```python
from build123d import *

# Parameters (mm, degrees)
SKETCH1_R           = 46.5
SKETCH1_R_2         = 36
BOSS_EXTRUDE1_DEPTH = 6.25
SKETCH4_R           = 36
SKETCH4_R_2         = 34
BOSS_EXTRUDE2_DEPTH = 3.5
SKETCH3_R           = 1.75
CUT_EXTRUDE1_DEPTH  = 67.938404522
CIRPATTERN1_COUNT   = 8


with BuildPart() as part:
    # Sketch1 → Boss-Extrude1 (new, symmetric)
    with BuildSketch(Plane.XY):
        Circle(SKETCH1_R)
        Circle(SKETCH1_R_2, mode=Mode.SUBTRACT)
    extrude(amount=BOSS_EXTRUDE1_DEPTH, both=True)

    # Sketch4 → Boss-Extrude2 (add)
    with BuildSketch(Plane.XY.offset(-6.25)):
        Circle(SKETCH4_R)
        Circle(SKETCH4_R_2, mode=Mode.SUBTRACT)
    extrude(amount=BOSS_EXTRUDE2_DEPTH)

    # Sketch3 → Cut-Extrude1 (cut, through all)
    with BuildSketch(Plane.XY.offset(6.25)):
        with Locations((0, 40.25)):
            Circle(SKETCH3_R)
    cut_extrude1 = extrude(amount=-CUT_EXTRUDE1_DEPTH, mode=Mode.SUBTRACT)

    # CirPattern1: Cut-Extrude1 ×8 about axis
    cirpattern1_axis = Axis((0, 0, 0), (0, 0, 1))
    for i in range(1, CIRPATTERN1_COUNT):
        add(cut_extrude1.rotate(cirpattern1_axis, i * 360 / CIRPATTERN1_COUNT), mode=Mode.SUBTRACT)


solid = part.part
```
Work out the finished part from the listing and answer in its coordinate system (mm). A direction names the side the tool comes from. Coordinates: 2 decimals unless noted, no trailing zeros. Write each loop counter-clockwise with the first axis right and the second up, starting at its lowest first coordinate (ties: lowest second). Pieces come first, ordered by that corner, then holes. Notation, with made-up numbers: (60.25, -11.5) - (116.25, -11.5) arc R15 ccw to (116.25, 13.5) - close; hole circle Ø2 at (-16.5, -11.75). An arc over 180 degrees is marked (long way). Answer as a JSON object with one key per item and string values.
Q1. Which of the six approach directions +Z, -Z, +X, -X, +Y, -Y give full straight-line access (tool end or side, diameter ignored) to faces 1 (the cylindrical face through (-26.792, 27.934, 0.088)), 2 (the cylindrical face through (-4.686, 35.694, 1.687))?
Results list:
{"face 1": "+Z, -Z", "face 2": "+Z"}
Q2. For a pull along Y with two mould halves and no side action, classify faces 3 (the cylindrical face through (26.792, -27.934, 0.088)), 4 (the cylindrical face through (44.35, 13.97, 0.09)), 5 (the flat face through (-4, -34, -6.25)), 6 (the cylindrical face through (-27.934, -26.792, 0.088)) as pulls with the +Y half, pulls with the -Y half, needs draft (parallel to the pull), parting line crosses it, or undercut.
Results list:
{"face 3": "undercut", "face 4": "parting line crosses it", "face 5": "needs draft", "face 6": "undercut"}
Q3. Given pin 1 Ø5.5 at (x, y) = (28.46, 28.46) entering from -Z; pin 2 Ø5 at (x, z) = (14, 1.5) entering from +Y; pin 3 Ø3 at (x, y) = (28.46, -28.46) entering from +Z; pin 4 Ø2 at (y, z) = (23, 3) entering from -X, each flat-ended and moving along its own axis, determine where each tip first touches the part or whether it passes through.
Results list:
{"pin 1": "stops at z = -6.25", "pin 2": "stops at y = 45.06", "pin 3": "passes through", "pin 4": "stops at x = -40.97"}
Q4. Consider L1, parallel to Y at x = 0, z = 4.25; L2, parallel to X at y = -33, z = -0.75; L3, parallel to Y at x = -12.5, z = -4.75. Determine where each line is inside the solid, lowest interval first. Write a range as from..to.
Results list:
{"L1": "y = -46.5..-42, -38.5..-36, 36..38.5, 42..46.5", "L2": "x = -32.76..-14.39, 14.39..32.76", "L3": "y = -44.79..-31.62, 31.62..44.79"}
Q5. Find section D-D (z = 1). State how many separate pieces and enclosed holes the cut face has, plus the area to 3 significant figures.
Results list:
{"separate pieces": "1", "enclosed holes": "9", "area": "2,640 mm^2"}
Q6. Find section A-A (y = 0). Write down the section's boundary in (x, z), plus the area to 3 significant figures.
Results list:
{"outline": "(-46.5, -6.25) - (-42, -6.25) - (-42, 6.25) - (-46.5, 6.25) - close; (-38.5, -6.25) - (-34, -6.25) - (-34, -2.75) - (-36, -2.75) - (-36, 6.25) - (-38.5, 6.25) - close; (34, -6.25) - (38.5, -6.25) - (38.5, 6.25) - (36, 6.25) - (36, -2.75) - (34, -2.75) - close; (42, -6.25) - (46.5, -6.25) - (46.5, 6.25) - (42, 6.25) - close", "area": "189 mm^2"}
Q7. Find section B-B (x = -20). Write down the section's boundary in (y, z), plus the area to 3 significant figures.
Results list:
{"outline": "(-41.98, -6.25) - (-27.5, -6.25) - (-27.5, -2.75) - (-29.93, -2.75) - (-29.93, 6.25) - (-41.98, 6.25) - close; (27.5, -6.25) - (41.98, -6.25) - (41.98, 6.25) - (29.93, 6.25) - (29.93, -2.75) - (27.5, -2.75) - close", "area": "318 mm^2"}
Q8. Find section C-C (y = -40.25). Write down the section's boundary in (x, z), plus the area to 3 significant figures.
Results list:
{"outline": "(-23.28, -6.25) - (-1.75, -6.25) - (-1.75, 6.25) - (-23.28, 6.25) - close; (1.75, -6.25) - (23.28, -6.25) - (23.28, 6.25) - (1.75, 6.25) - close", "area": "538 mm^2"}
